Part model, mm, in its own coordinate system. A direction names the side the tool comes from. Round coordinates to 2 decimals unless told otherwise and drop trailing zeros. Write each loop counter-clockwise with the first axis right and the second up, starting at its lowest first coordinate (ties: lowest second). Pieces come first, ordered by that corner, then holes. Notation, with made-up numbers: (39.25, 7) -> (48.25, 7) arc R23 ccw to (48.25, 23) -> close; hole circle Ø2 at (40, -34). An arc over 180 degrees is marked (long way). Return JSON: item names as keys, results as strings. Group by question number.
```python
from build123d import *

# Parameters (mm, degrees)
ESBO_O1_R                 = 24
ESBO_O1_R_2               = 6
RESSALTO_EXTRUS_O1_DEPTH  = 5
ESBO_O2_R                 = 2.5
CORTE_EXTRUS_O1_DEPTH     = 45.905785333
CORTE_EXTRUS_O2_START     = -5
CORTE_EXTRUS_O2_OUTLINE_R = 2.5
CORTE_EXTRUS_O2_DEPTH     = 5


# Read off the part's stored shape, not the designer's step: Corte-extrusão2
with BuildPart() as part:
    # Esboço1 → Ressalto-extrusão1 (new body)
    with BuildSketch(Plane.XY):
        with Locations((4.905528128, 10)):
            Circle(ESBO_O1_R)
        with Locations((4.905528128, 10)):
            Circle(ESBO_O1_R_2, mode=Mode.SUBTRACT)
    extrude(amount=RESSALTO_EXTRUS_O1_DEPTH)

    # Esboço2 → Corte-extrusão1 (cut, through all)
    with BuildSketch(Plane.XY.offset(5)):
        with Locations((4.905528128, 28)):
            Circle(ESBO_O2_R)
        with Locations((20.493985396, 19)):
            Circle(ESBO_O2_R)
        with Locations((20.493985396, 1)):
            Circle(ESBO_O2_R)
        with Locations((4.905528128, -8)):
            Circle(ESBO_O2_R)
        with Locations((-10.68292914, 1)):
            Circle(ESBO_O2_R)
        with Locations((-10.68292914, 19)):
            Circle(ESBO_O2_R)
    extrude(amount=-CORTE_EXTRUS_O1_DEPTH, mode=Mode.SUBTRACT)

    # Corte-extrusão2 outline → Corte-extrusão2 (cut)
    # profile 1 of 3: a face of its own
    with BuildSketch(Plane.XY.offset(5).offset(CORTE_EXTRUS_O2_START)):
        with BuildLine():
            ThreePointArc((4.897969025, 21.999997619), (4.901748576, 21.999999405), (4.905528128, 22))
            ThreePointArc((4.905528128, 22), (11.295284197, 22.550508098), (17.493985396, 24.196152423))
            ThreePointArc((17.493985396, 24.196152423), (22.046899667, 24.795554958), (25.690137819, 22))
            ThreePointArc((25.690137819, 22), (4.905528128, 34), (-15.879081563, 22))
            ThreePointArc((-15.879081563, 22), (-12.235843411, 24.795554958), (-7.68292914, 24.196152423))
            ThreePointArc((-7.68292914, 24.196152423), (-1.487951224, 22.551157849), (4.897969025, 21.999997619))
        make_face()
        with Locations((4.905528128, 28)):
            Circle(CORTE_EXTRUS_O2_OUTLINE_R, mode=Mode.SUBTRACT)
    # profile 2 of 3: a face of its own
    with BuildSketch(Plane.XY.offset(5).offset(CORTE_EXTRUS_O2_START)):
        with BuildLine():
            ThreePointArc((4.905528128, -14), (25.690137819, -2), (25.690137819, 22))
            ThreePointArc((25.690137819, 22), (26.289540354, 17.447085729), (23.493985396, 13.803847577))
            ThreePointArc((23.493985396, 13.803847577), (18.971889348, 9.261336613), (15.301607732, 4.006549141))
            ThreePointArc((15.301607732, 4.006549141), (15.299722234, 4.003273486), (15.297832974, 4))
            ThreePointArc((15.297832974, 4), (12.579708936, -1.808945129), (10.905528128, -8))
            ThreePointArc((10.905528128, -8), (9.148168815, -12.242640687), (4.905528128, -14))
        make_face()
        with Locations((20.493985396, 1)):
            Circle(CORTE_EXTRUS_O2_OUTLINE_R, mode=Mode.SUBTRACT)
    # profile 3 of 3: a face of its own
    with BuildSketch(Plane.XY.offset(5).offset(CORTE_EXTRUS_O2_START)):
        with BuildLine():
            ThreePointArc((-13.68292914, 13.803847577), (-16.478484098, 17.447085729), (-15.879081563, 22))
            ThreePointArc((-15.879081563, 22), (-15.879081563, -2), (4.905528128, -14))
            ThreePointArc((4.905528128, -14), (0.662887441, -12.242640687), (-1.094471872, -8))
            ThreePointArc((-1.094471872, -8), (-2.76865268, -1.808945129), (-5.486776717, 4))
            ThreePointArc((-5.486776717, 4), (-5.488665978, 4.003273485), (-5.490554207, 4.006547566))
            ThreePointArc((-5.490554207, 4.006547566), (-9.160833092, 9.261336613), (-13.68292914, 13.803847577))
        make_face()
        with Locations((-10.68292914, 1)):
            Circle(CORTE_EXTRUS_O2_OUTLINE_R, mode=Mode.SUBTRACT)
    extrude(amount=CORTE_EXTRUS_O2_DEPTH, mode=Mode.SUBTRACT)


solid = part.part
```
Item 1: Cut at B-B (x = -12). Write the cut outline in (y, z).
Item 2: Flat gauge pins, fed straight in: P1, Ø8, axis at x = 4.91, y = -8, coming from the -Z side; P2, Ø2, axis at x = 2, z = 2, coming from the -Y side; P3, Ø4, axis at x = -10.68, y = 19, coming from the -Z side; P4, Ø1, axis at x = 8.5, z = 4, coming from the -Y side. Where does each tip first touch, or does it go through?
Item 3: Cut at C-C (z = 0.8). State how many separate pieces and enclosed holes the cut face has, then the cut area to 3 significant figures.
Item 4: Which spindle directions (+Z, -Z, +X, -X, +Y, -Y) get a long thin tool onto all of the face, cutting with end or side? Do faces 1 (the face through (-1.576, 22.567, 2.465)), 2 (the face through (-9.1, 9.19, 2.46)). Say none if no direction does.
Item 5: Cut at D-D (y = 5). Write the cut outline in (x, z).
Item 6: Wall check: L1, parallel to X at y = 21, z = 3.9; L2, parallel to Y at x = -10.5, z = 1.9; L3, parallel to X at y = -6, z = 1.95. Give the ranges that are in metal, low to high.
Item 7: Two-plate mould, pull along X, no slides. Class faces 3 (the face through (-9.34, 21.11, 2.54)), 4 (the face through (-2.74, -1.89, 2.46)), 5 (the face through (3.605, 4.143, 2.465)), 6 (the face through (9.4, 14.4, 0)): released by +X, released by -X, zero draft, split by the parting line, or undercut.
Item 8: Cut at A-A (y = 19). Write the cut outline in (x, z), then the cut area to 3 significant figures.
Checks:
{
 "1": {"outline": "(12.29, 0) -> (16.88, 0) -> (16.88, 5) -> (12.29, 5) -> close; (21.12, 0) -> (24.85, 0) -> (24.85, 5) -> (21.12, 5) -> close"},
 "2": {"P1": "stops at z = 0", "P2": "stops at y = -13.69", "P3": "passes through", "P4": "stops at y = -13.14"},
 "3": {"separate pieces": "1", "enclosed holes": "4", "area": "746 mm2"},
 "4": {"face 1": "+Z, -Z, +Y", "face 2": "+Z, -Z, -X, -Y"},
 "5": {"outline": "(-6.08, 0) -> (1.59, 0) -> (1.59, 5) -> (-6.08, 5) -> close; (8.22, 0) -> (15.9, 0) -> (15.9, 5) -> (8.22, 5) -> close"},
 "6": {"L1": "x = -16.34 to -12.18, -9.18 to 18.99, 21.99 to 26.15", "L2": "y = 10.78 to 16.51, 21.49 to 25", "L3": "x = -1.51 to 3.41, 6.41 to 11.32"},
 "7": {"face 3": "undercut", "face 4": "released by -X", "face 5": "undercut", "face 6": "zero draft"},
 "8": {"outline": "(-16.68, 0) -> (-13.18, 0) -> (-13.18, 5) -> (-16.68, 5) -> close; (-8.18, 0) -> (17.99, 0) -> (17.99, 5) -> (-8.18, 5) -> close; (22.99, 0) -> (26.49, 0) -> (26.49, 5) -> (22.99, 5) -> close", "area": "166 mm2"}
}
